from build123d import *

# Parameters (mm, degrees)
BOSS_EXTRUDE1_DEPTH = 6.477
FILLET1_R           = 1.905


with BuildPart() as part:
    # Sketch1 → Boss-Extrude1 (new body)
    with BuildSketch(Plane(origin=(0, 0, 0), x_dir=(0, 0, -1), z_dir=(1, 0, 0))):
        Polygon((-22.098, 0), (0, 0), (0, 3.048), (-19.05, 3.048), (-19.05, 9.398), (-22.098, 9.398), align=None)
    extrude(amount=BOSS_EXTRUDE1_DEPTH)

    # Fillet1
    fillet1_edges = [part.edges().sort_by_distance(p)[0] for p in [
        (6.477, 1.524, 0),
        (0, 1.524, 0),
    ]]
    fillet(fillet1_edges, radius=FILLET1_R)


solid = part.part
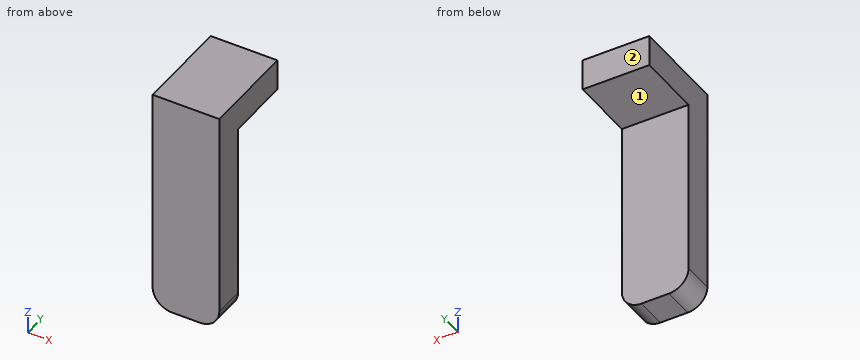
Geometry check sheet. Reference: the model listing, model coordinates, mm. Face numbers are marked on the shaded views. A direction names the side the tool comes from. Give positions to 0.01 mm unless a question says otherwise; leave off trailing zeros. Order: outer loops, then holes, each group sorted by start corner. A loop starts at its lowest first (then second) coordinate and runs counter-clockwise, first axis right, second up.
1) Tool access check on the marked faces 1 and 2. Record the directions out of +Z, -Z, +X, -X, +Y, -Y that give a thin tool (end or side, any length) a straight path to the whole face; none if there is none.
Results are:
face 1: -Z, +X, -X, +Y
face 2: +Z, -Z, +X, -X, +Y
2) Gauge pin test, flat ends, axial feed: pin 1 (3 mm diameter, centred on x = 3.5, z = 6, fed in from +Y); pin 2 (5 mm diameter, centred on y = 3.5, z = 19, fed in from -X); pin 3 (1.5 mm diameter, centred on x = 3.5, y = 7, fed in from -Z). Record the tip position at first contact, or that the pin passes through.
Results are:
pin 1: stops at y = 3.05
pin 2: stops at x = 0
pin 3: stops at z = 19.05
3) Cross-section at D-D (x = 1). Record the boundary of the cut face in (y, z), then the cut area to 3 significant figures.
Results are:
outline: (0, 0.23) - (3.05, 0.23) - (3.05, 19.05) - (9.4, 19.05) - (9.4, 22.1) - (0, 22.1) - close
area: 86.0 mm2
4) Material ranges on probe 1 along Z at (x, y) = (3, 5.25); probe 2 along Y at (x, z) = (1.5, 4), recorded low to high.
Results are:
probe 1: z = 19.05 to 22.1
probe 2: y = 0 to 3.05
5) Cross-section at A-A (x = 3). Record the boundary of the cut face in (y, z).
Results are:
outline: (0, 0) - (3.05, 0) - (3.05, 19.05) - (9.4, 19.05) - (9.4, 22.1) - (0, 22.1) - close
6) Cross-section at B-B (z = 9.75). Record the boundary of the cut face in (x, y).
Results are:
outline: (0, 0) - (6.48, 0) - (6.48, 3.05) - (0, 3.05) - close
7) Cross-section at C-C (y = 5.5). Record the boundary of the cut face in (x, z).
Results are:
outline: (0, 19.05) - (6.48, 19.05) - (6.48, 22.1) - (0, 22.1) - close
